from build123d import *

# Parameters (mm, degrees)
F0_R     = 4.7625
F1_DEPTH = 25.4
F3_DEPTH = 7.9375
F4_SIZE  = 0.254


with BuildPart() as f1:
    # F0 (on Front) → F1 (new body)
    with BuildSketch(Plane.XZ):
        Circle(F0_R)
    extrude(amount=F1_DEPTH)

    # F2 (on Front) → F3 (join)
    with BuildSketch(Plane.XZ):
        with BuildLine():
            ThreePointArc((-5.4992613166, 3.1749999956), (-3.1750000022, 5.4992613128), (0, 6.35))
            Line((0, 6.35), (-3.6661742094, 6.35))
            Line((-3.6661742094, 6.35), (-5.4992613166, 3.1749999956))
        make_face()
        with BuildLine():
            ThreePointArc((-5.499261351, -3.174999936), (-6.35, 3.44e-08), (-5.4992613166, 3.1749999956))
            Line((-5.4992613166, 3.1749999956), (-7.3323484187, 0))
            Line((-7.3323484187, 0), (-5.499261351, -3.174999936))
        make_face()
        with BuildLine():
            Line((-3.6661742094, -6.35), (0, -6.35))
            ThreePointArc((0, -6.35), (-3.175000032, -5.4992612955), (-5.499261351, -3.174999936))
            Line((-5.499261351, -3.174999936), (-3.6661742094, -6.35))
        make_face()
        with BuildLine():
            ThreePointArc((0, 6.35), (3.174999954, 5.4992613406), (5.4992612609, 3.175000092))
            Line((5.4992612609, 3.175000092), (3.6661742094, 6.35))
            Line((3.6661742094, 6.35), (0, 6.35))
        make_face()
        with BuildLine():
            ThreePointArc((5.4992612609, 3.175000092), (6.1336289832, 1.6435009877), (6.35, 0))
            ThreePointArc((6.35, 0), (6.1336290065, -1.6435009007), (5.499261351, -3.174999936))
            Line((5.499261351, -3.174999936), (7.3323484187, 0))
            Line((7.3323484187, 0), (5.4992612609, 3.175000092))
        make_face()
        with BuildLine():
            Line((3.6661742094, -6.35), (5.499261351, -3.174999936))
            ThreePointArc((5.499261351, -3.174999936), (3.175000032, -5.4992612955), (0, -6.35))
            Line((0, -6.35), (3.6661742094, -6.35))
        make_face()
        with BuildLine():
            ThreePointArc((5.499261351, -3.174999936), (6.1336290065, -1.6435009007), (6.35, 0))
            ThreePointArc((6.35, 0), (6.1336289832, 1.6435009877), (5.4992612609, 3.175000092))
            ThreePointArc((5.4992612609, 3.175000092), (3.174999954, 5.4992613406), (0, 6.35))
            ThreePointArc((0, 6.35), (-3.1750000022, 5.4992613128), (-5.4992613166, 3.1749999956))
            ThreePointArc((-5.4992613166, 3.1749999956), (-6.35, 3.44e-08), (-5.499261351, -3.174999936))
            ThreePointArc((-5.499261351, -3.174999936), (-3.175000032, -5.4992612955), (0, -6.35))
            ThreePointArc((0, -6.35), (3.175000032, -5.4992612955), (5.499261351, -3.174999936))
        make_face()
    extrude(amount=F3_DEPTH)

    # F4
    f4_edges = [f1.edges().sort_by_distance(p)[0] for p in [
        (-4.7625, -25.4, 0),
    ]]
    chamfer(f4_edges, length=F4_SIZE)


solid = f1.part
Can you work these out from the model? Positions are in its coordinate system, mm. A direction names the side the tool comes from. Give positions to 0.01 mm unless a question says otherwise; leave off trailing zeros. Loops run counter-clockwise (first coordinate to the right, second up) from the corner with the lowest first, then second, coordinate; pieces in that order, holes last. Notation, with made-up numbers: M -39,-9 L -10,-9 A12 cw -10,12 Z; hole C 63,46 d5. An arc over 180 degrees is marked long. One line per item, written item: value. Start each with the question number.
1) I'm going to push flat-ended pins straight in: pin 1 (4 mm diameter, centred on x = 2, y = -8.5, fed in from -Z); pin 2 (3 mm diameter, centred on y = -3.5, z = 2.5, fed in from -X) (3 decimals); pin 3 (2 mm diameter, centred on x = -4.5, z = -3.5, fed in from -Y); pin 4 (1.5 mm diameter, centred on y = -14.5, z = -3, fed in from +X). Where does each tip first touch, or does it pass through?
2) If we section it at B-B, the plane y = -21.5: Write out the boundary of the cut face in (x, z) (1 decimal), and give its area (3 significant figures).
3) If we section it at A-A, the plane x = 0: Write out the boundary of the cut face in (y, z), and give its area (3 significant figures).
4) On a 3-axis mill with a long thin cutter (end or side, diameter ignored), from which of +Z, -Z, +X, -X, +Y, -Y can I reach the whole of each face in a straight line? I mean faces 1 (the face through (0, -4, 6.35)), 2 (the face through (5, -7.938, 0)). Say none if no direction works.
5) If I drill on line 1 (Y direction, x = 5, z = 0.5); line 2 (X direction, y = -4.5, z = 1.5); line 3 (X direction, y = -10.5, z = -3), over which ranges is the centre line in solid material (lowest first)? Write a range as [from, to].
Completed:
1. pin 1: stops at z = -6.35
1. pin 2: stops at x = -6.755
1. pin 3: stops at y = -25.21
1. pin 4: stops at x = 4.2
2. outline: C 0,0 d9.5
2. area: 71.3 mm^2
3. outline: M -25.4,-4.51 L -25.15,-4.76 L -7.94,-4.76 L -7.94,-6.35 L 0,-6.35 L 0,6.35 L -7.94,6.35 L -7.94,4.76 L -25.15,4.76 L -25.4,4.51 Z
3. area: 267 mm^2
4. face 1: +Z, +X, -X, +Y, -Y
4. face 2: -Y
5. line 1: y = [-7.94, 0]
5. line 2: x = [-6.47, 6.47]
5. line 3: x = [-3.7, 3.7]
